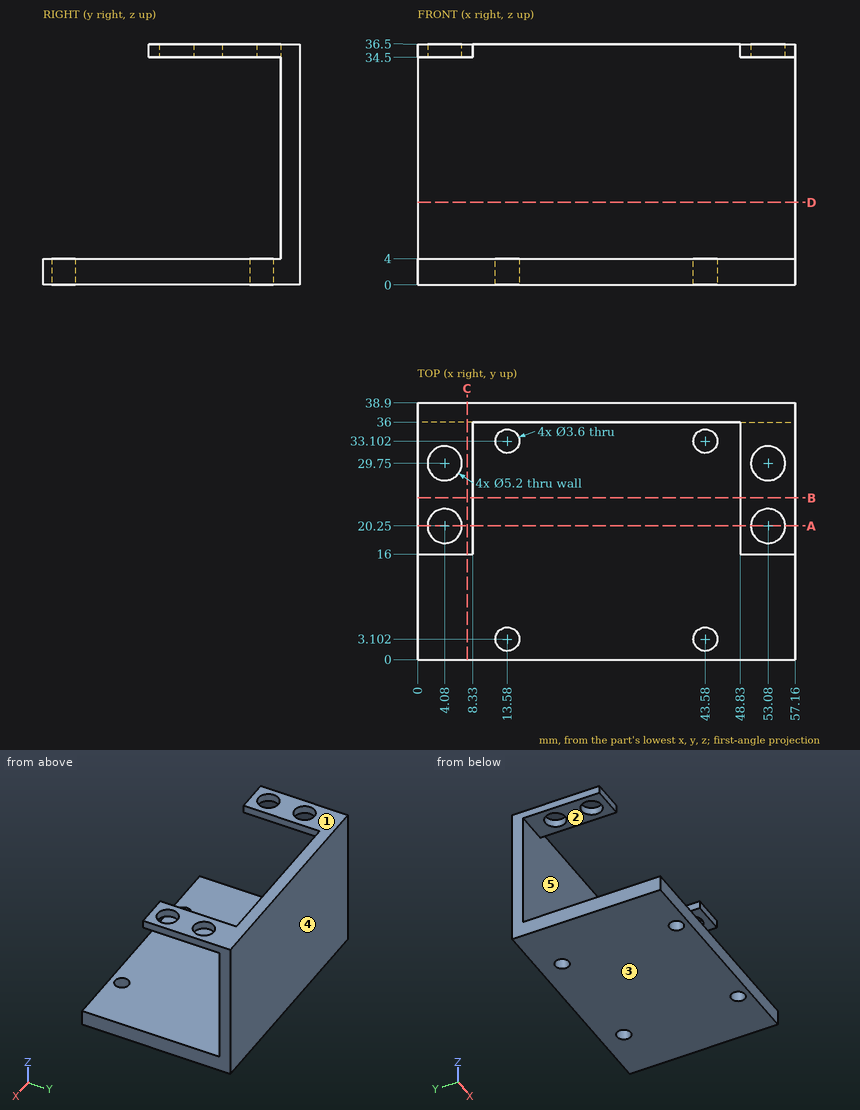
Here's the drawing with two shaded views (mm, measured from the low corner). I have some questions. A direction names the side the tool comes from. Coordinates: 2 decimals unless noted, no trailing zeros. Order: outer loops, then holes, each group sorted by start corner. A loop starts at its lowest first (then second) coordinate and runs counter-clockwise, first axis right, second up. Notation, with made-up numbers: (58, 88.25) - (75, 88.25) arc R14 cw to (75, 111.25) - close; hole circle Ø1 at (73.25, -10). An arc over 180 degrees is marked (long way). Answer in a Markdown table with one row per item.
1. If we mould it in two halves opening along Z, with no side actions, what happens to the marked faces 3, 4 and 5? For each: pulls with the +Z half, pulls with the -Z half, needs draft (parallel to the pull), parting line crosses it, or undercut.
Reply:
| item | result |
|---|---|
| face 3 | pulls with the -Z half |
| face 4 | needs draft |
| face 5 | undercut |
2. Suppose I cut it at D-D (z = 12.5). Please give me the cut outline in (x, y), and give its area (3 significant figures).
Reply:
| item | result |
|---|---|
| outline | (0, 36) - (57.16, 36) - (57.16, 38.9) - (0, 38.9) - close |
| area | 166 mm^2 |
3. Suppose I cut it at B-B (y = 24.5). Please give me the cut outline in (x, z), and give its area (3 significant figures).
Reply:
| item | result |
|---|---|
| outline | (0, 0) - (57.16, 0) - (57.16, 4) - (0, 4) - close; (0, 34.5) - (8.33, 34.5) - (8.33, 36.5) - (0, 36.5) - close; (48.83, 34.5) - (57.16, 34.5) - (57.16, 36.5) - (48.83, 36.5) - close |
| area | 262 mm^2 |
4. Suppose I cut it at C-C (x = 7.5). Please give me the cut outline in (y, z).
Reply:
| item | result |
|---|---|
| outline | (0, 0) - (38.9, 0) - (38.9, 36.5) - (16, 36.5) - (16, 34.5) - (36, 34.5) - (36, 4) - (0, 4) - close |
5. If I drill on line 1 along Y through (x, z) = (9.5, 28.5); line 2 along Z through (x, y) = (23.5, 4), over which ranges is the centre line in solid material (lowest first)?
Reply:
| item | result |
|---|---|
| line 1 | y = 36 to 38.9 |
| line 2 | z = 0 to 4 |
6. Suppose I cut it at A-A (y = 20.25). Please give me the cut outline in (x, z), and give its area (3 significant figures).
Reply:
| item | result |
|---|---|
| outline | (0, 0) - (57.16, 0) - (57.16, 4) - (0, 4) - close; (0, 34.5) - (1.48, 34.5) - (1.48, 36.5) - (0, 36.5) - close; (6.68, 34.5) - (8.33, 34.5) - (8.33, 36.5) - (6.68, 36.5) - close; (48.83, 34.5) - (50.48, 34.5) - (50.48, 36.5) - (48.83, 36.5) - close; (55.68, 34.5) - (57.16, 34.5) - (57.16, 36.5) - (55.68, 36.5) - close |
| area | 241 mm^2 |
7. For the marked faces 1 and 2, which set-ups out of +Z, -Z, +X, -X, +Y, -Y let a thin tool reach every point of the face, with its end or its side?
Reply:
| item | result |
|---|---|
| face 1 | +Z, +X, -X, +Y, -Y |
| face 2 | +X, -X, -Y |
8. For pin 1 (0.6 mm diameter, centred on x = 54.5, z = 36, fed in from -Y); pin 2 (6 mm diameter, centred on x = 13.5, z = 19.5, fed in from -Y); pin 3 (3 mm diameter, centred on x = 43.58, y = 3.1, fed in from +Z); pin 4 (18 mm diameter, centred on x = 24.5, y = 18.5, fed in from +Z), each with a flat end and sliding along its axis, tell me the tip position at first contact or that it passes through.
Reply:
| item | result |
|---|---|
| pin 1 | stops at y = 16 |
| pin 2 | stops at y = 36 |
| pin 3 | passes through |
| pin 4 | stops at z = 4 |
